from build123d import *

# Parameters (mm, degrees)
F1_DEPTH = 100
F3_D     = 5.5
F5_D     = 4.2
F5_DEPTH = 14.4
F5_TIP   = 1.2618073


with BuildPart() as f1:
    # F0 (on Right) → F1 (new body)
    with BuildSketch(Plane.YZ):
        Polygon((-120, 0), (0, 0), (0, 10), (-10, 10), (-120, 10), align=None)
    extrude(amount=F1_DEPTH)

    # F3 (through all)
    with Locations(Plane.XY.offset(10)):
        with Locations((80, -10), (80, -42), (20, -42), (20, -10), (39, -70), (61, -70), (61, -110), (39, -110)):
            Hole(F3_D / 2)

    # F5
    with Locations(Plane(origin=(0, 0, 0), x_dir=(-1, 0, 0), z_dir=(0, 1, 0))):
        with Locations((-90, 5), (-65, 5), (-35, 5), (-10, 5)):
            Hole(F5_D / 2, depth=F5_DEPTH)
            with Locations((0, 0, -(F5_DEPTH + F5_TIP / 2))):  # 118° drill point
                Cone(0, F5_D / 2, F5_TIP, mode=Mode.SUBTRACT)


solid = f1.part
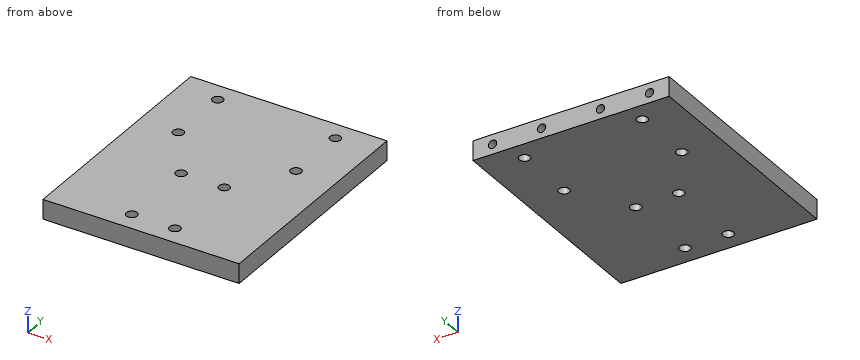
Could you check a few things on this model? Use its own coordinates, in mm. Coordinates: 2 decimals unless noted, no trailing zeros. Loops run counter-clockwise (first coordinate to the right, second up) from the corner with the lowest first, then second, coordinate; pieces in that order, holes last.
1. Imagine slicing it at B-B (x = 80). Please give me the cut outline in (y, z).
2. Imagine slicing it at C-C (y = -70). Please give me the cut outline in (x, z).
3. I need wall thicknesses on L1, parallel to Y at x = 80, z = 7; L2, parallel to Y at x = 61, z = 4; L3, parallel to Z at x = 10, y = -10. Which ranges of each line are inside material? Lowest first, please.
4. Imagine slicing it at A-A (z = 8.5). Give the number of separate pieces and of enclosed holes in the cut face, and give its area (3 significant figures).
Computed values:
1. outline: (-120, 0) - (-44.75, 0) - (-44.75, 10) - (-120, 10) - close; (-39.25, 0) - (-12.75, 0) - (-12.75, 10) - (-39.25, 10) - close; (-7.25, 0) - (0, 0) - (0, 10) - (-7.25, 10) - close
2. outline: (0, 0) - (36.25, 0) - (36.25, 10) - (0, 10) - close; (41.75, 0) - (58.25, 0) - (58.25, 10) - (41.75, 10) - close; (63.75, 0) - (100, 0) - (100, 10) - (63.75, 10) - close
3. L1: y = -120 to -44.75, -39.25 to -12.75, -7.25 to 0
3. L2: y = -120 to -112.75, -107.25 to -72.75, -67.25 to 0
3. L3: z = 0 to 2.9, 7.1 to 10
4. separate pieces: 1
4. enclosed holes: 8
4. area: 11,800 mm2
